Can you work these out from the model? Positions are in its coordinate system, mm. A direction names the side the tool comes from. Round coordinates to 2 decimals unless told otherwise and drop trailing zeros. Order: outer loops, then holes, each group sorted by start corner. A loop starts at its lowest first (then second) coordinate and runs counter-clockwise, first axis right, second up. Notation, with made-up numbers: (-23.75, 27) -> (-16.75, 27) arc R20 cw to (-16.75, 39) -> close; hole circle Ø2 at (65, 4.25). An arc over 180 degrees is marked (long way). One line per item, written item: value.
```python
from build123d import *
from OCP.BRepFilletAPI import BRepFilletAPI_MakeChamfer

# Parameters (mm, degrees)
SKETCH_2_W          = 20.5
SKETCH_2_H          = 12
EXTRUDE_1_DEPTH     = 30
SKETCH_3_W          = 22
SKETCH_3_H          = 4.27428741
CUT_EXTRUDE_1_DEPTH = 34.897824414
SKETCH_10_W         = 17.106520138
SKETCH_10_H         = 9.063555791
CUT_EXTRUDE_3_DEPTH = 34.897824414
SKETCH_11_R         = 1.5
CUT_EXTRUDE_6_DEPTH = 35.706461629
SKETCH_12_R         = 0.75
CUT_EXTRUDE_4_DEPTH = 12
CUT_EXTRUDE_7_DEPTH = 37.827299657
CHAMFER_5_SIZE      = 2
CHAMFER_6_SIZE      = 2
CHAMFER_6_SIZE2     = 2.003351387
SKETCH_14_R         = 0.75
CUT_EXTRUDE_5_DEPTH = 23.406751215
CHAMFER_8_SIZE      = 3
CUT_EXTRUDE_8_DEPTH = 10


with BuildPart() as part:
    # Эскиз2 → Вытянуть1 (new body)
    with BuildSketch(Plane(origin=(0, 0, 0), x_dir=(0, 0, -1), z_dir=(1, 0, 0))):
        Rectangle(SKETCH_2_W, SKETCH_2_H)
    extrude(amount=EXTRUDE_1_DEPTH)

    # Эскиз3 → Вырез-Вытянуть1 (cut, through all)
    with BuildSketch(Plane(origin=(0, 6, 0), x_dir=(1, 0, 0), z_dir=(0, 1, 0))):
        Rectangle(SKETCH_3_W, SKETCH_3_H)
    extrude(amount=-CUT_EXTRUDE_1_DEPTH, mode=Mode.SUBTRACT)

    # Эскиз10 → Вырез-Вытянуть3 (cut, through all)
    with BuildSketch(Plane(origin=(0, 6, 0), x_dir=(1, 0, 0), z_dir=(0, 1, 0))):
        with Locations((2.446739931, 10.668921601)):
            Rectangle(SKETCH_10_W, SKETCH_10_H)
        with Locations((2.446739931, -10.668921601)):
            Rectangle(SKETCH_10_W, SKETCH_10_H)
    extrude(amount=-CUT_EXTRUDE_3_DEPTH, mode=Mode.SUBTRACT)

    # Эскиз11 → Вытянуть6 (cut, through all)
    with BuildSketch(Plane.XY.offset(6.137143705)):
        with Locations((4.5, -1.5)):
            Circle(SKETCH_11_R)
    extrude(amount=-CUT_EXTRUDE_6_DEPTH, mode=Mode.SUBTRACT)

    # Эскиз12 → Вырез-Вытянуть4 (cut)
    with BuildSketch(Plane.ZY.offset(-11)):
        with Locations((-1.791386219, -3.407348241)):
            Circle(SKETCH_12_R)
    extrude(amount=-CUT_EXTRUDE_4_DEPTH, mode=Mode.SUBTRACT)

    # Эскиз13 → Вытянуть7 (cut, through all)
    with BuildSketch(Plane.XY.offset(10.25)):
        Polygon((10.95, 6), (0, 6), (0, 2), align=None)
        Polygon((40.005782236, 6), (40.005782236, 2), (30.005782236, 6), align=None)
    extrude(amount=-CUT_EXTRUDE_7_DEPTH, mode=Mode.SUBTRACT)

    # Фаска5
    chamfer_5_edges = [part.edges().sort_by_distance(p)[0] for p in [
        (30, -6, 0),
        (0, -6, -4.137143705),
        (0, -6, 4.137143705),
        (30, 6, 0),
    ]]
    chamfer(chamfer_5_edges, length=CHAMFER_5_SIZE)

    # Фаска6: one chamfer whose edges measure the first distance from different faces: ONE call of the kernel's chamfer builder (chamfer() names one face for all edges)
    chamfer_6_edges_1 = [part.edges().sort_by_distance(p)[0] for p in [
        (0, 2, 4.137143705),
    ]]
    chamfer_6_side_1 = [part.faces().sort_by_distance(p)[0] for p in [
        (0, -1, 4.137143705),
    ]]
    chamfer_6_edges_2 = [part.edges().sort_by_distance(p)[0] for p in [
        (0, 2, -4.137143705),
    ]]
    chamfer_6_side_2 = [part.faces().sort_by_distance(p)[0] for p in [
        (0, -1, -4.137143705),
    ]]
    chamfer_6 = BRepFilletAPI_MakeChamfer(part.part.solid().wrapped)
    for e in chamfer_6_edges_1:
        chamfer_6.Add(CHAMFER_6_SIZE, CHAMFER_6_SIZE2, e.wrapped, chamfer_6_side_1[0].wrapped)  # the first distance lies on this face
    for e in chamfer_6_edges_2:
        chamfer_6.Add(CHAMFER_6_SIZE, CHAMFER_6_SIZE2, e.wrapped, chamfer_6_side_2[0].wrapped)  # the first distance lies on this face
    add(Compound.cast(chamfer_6.Shape()), mode=Mode.REPLACE)

    # Эскиз14 → Вырез-Вытянуть5 (cut, through all)
    with BuildSketch(Plane.ZY.offset(-11)):
        with Locations((0, 3.465363476)):
            Circle(SKETCH_14_R)
    extrude(amount=-CUT_EXTRUDE_5_DEPTH, mode=Mode.SUBTRACT)

    # Фаска8
    chamfer_8_edges = [part.edges().sort_by_distance(p)[0] for p in [
        (11, 6, -8.193571852),
        (11, 6, 8.193571852),
    ]]
    chamfer(chamfer_8_edges, length=CHAMFER_8_SIZE)

    # Эскиз15 → Вытянуть8 (cut)
    with BuildSketch(Plane.XZ.offset(6)):
        with BuildLine():
            Line((16, 6.25), (25, 6.25))
            ThreePointArc((25, 6.25), (26.414213562, 5.664213562), (27, 4.25))
            Line((27, 4.25), (27, -4.25))
            ThreePointArc((27, -4.25), (26.414213562, -5.664213562), (25, -6.25))
            Line((25, -6.25), (16, -6.25))
            ThreePointArc((16, -6.25), (14.585786438, -5.664213562), (14, -4.25))
            Line((14, -4.25), (14, 4.25))
            ThreePointArc((14, 4.25), (14.585786438, 5.664213562), (16, 6.25))
        make_face()
    extrude(amount=-CUT_EXTRUDE_8_DEPTH, mode=Mode.SUBTRACT)


solid = part.part
```
Q1. I want a section at C-C on x = 17.75. List the corners of the cut face in (y, z) for me, plus the area to 3 significant figures.
Answers below:
outline: (-6, -10.25) -> (6, -10.25) -> (6, 10.25) -> (-6, 10.25) -> (-6, 6.25) -> (4, 6.25) -> (4, 0.53) arc R0.75 cw to (4, -0.53) -> (4, -6.25) -> (-6, -6.25) -> close
area: 121 mm^2
Q2. Please list where these lines run through material, in increasing order: line 1 along X through (y, z) = (-1.5, 1.5); line 2 along Z through (x, y) = (20.5, -0.75); line 3 along Z through (x, y) = (5.5, 2).
Answers below:
line 1: 11 to 14, 27 to 30
line 2: -10.25 to -6.25, 6.25 to 10.25
line 3: -6.14 to -2.14, 2.14 to 6.14
Q3. I want a section at B-B on z = 0. List the corners of the cut face in (x, y) for me, plus the area to 3 significant figures.
Answers below:
outline: (11, -6) -> (14, -6) -> (14, 2.72) -> (11, 2.72) -> close; (11, 4.22) -> (29.78, 4.22) -> (28, 6) -> (11, 6) -> close; (27, -6) -> (28, -6) -> (30, -4) -> (30, 2.72) -> (27, 2.72) -> close
area: 82.2 mm^2
Q4. I want a section at D-D on y = -4.5. List the corners of the cut face in (x, z) for me, plus the area to 3 significant figures.
Answers below:
outline: (0.5, -6.14) -> (11, -6.14) -> (11, -10.25) -> (29.5, -10.25) -> (29.5, 10.25) -> (11, 10.25) -> (11, 6.14) -> (0.5, 6.14) -> (0.5, 2.14) -> (11, 2.14) -> (11, -2.14) -> (0.5, -2.14) -> close; hole (14, -4.25) arc R2 ccw to (16, -6.25) -> (25, -6.25) arc R2 ccw to (27, -4.25) -> (27, 4.25) arc R2 ccw to (25, 6.25) -> (16, 6.25) arc R2 ccw to (14, 4.25) -> close
area: 304 mm^2
Q5. We'd pull the mould along X, two halves only. Please class faces 1 (the face through (12, 4, -8)), 2 (the face through (30, 0, 0)), 3 (the face through (5.886, -2.075, -4.109)): released by +X, released by -X, zero draft, split by the parting line, or undercut.
Answers below:
face 1: released by -X
face 2: released by +X
face 3: undercut
Q6. On a 3-axis mill with a long thin cutter (end or side, diameter ignored), from which of +Z, -Z, +X, -X, +Y, -Y can I reach the whole of each face in a straight line? I mean faces 4 (the face through (7, -1, 2.137)), 5 (the face through (12, 4, 8)), 6 (the face through (26.4, -1.07, 5.68)). Say none if no direction works.
Answers below:
face 4: -X, +Y, -Y
face 5: +Z, -X, +Y
face 6: -Y
Q7. Will these pins go through, and if not, where does the flat tip stop? pin 1 Ø1.2 at (y, z) = (0.5, -8.5) entering from -X; pin 2 Ø6 at (x, y) = (4, 1) entering from +Z; pin 3 Ø2 at (x, z) = (17, 3.5) entering from -Y.
Answers below:
pin 1: x = 11
pin 2: z = 6.14
pin 3: y = 4
Q8. I want a section at A-A on y = -1.5. List the corners of the cut face in (x, z) for me.
Answers below:
outline: (0, -6.14) -> (3, -6.14) -> (3, -2.14) -> (0, -2.14) -> close; (0, 2.14) -> (3, 2.14) -> (3, 6.14) -> (0, 6.14) -> close; (6, -6.14) -> (11, -6.14) -> (11, -10.25) -> (30, -10.25) -> (30, 10.25) -> (11, 10.25) -> (11, 6.14) -> (6, 6.14) -> (6, 2.14) -> (11, 2.14) -> (11, -2.14) -> (6, -2.14) -> close; hole (14, -4.25) arc R2 ccw to (16, -6.25) -> (25, -6.25) arc R2 ccw to (27, -4.25) -> (27, 4.25) arc R2 ccw to (25, 6.25) -> (16, 6.25) arc R2 ccw to (14, 4.25) -> close
